Check sheet for the modelled part. Datum: model origin and axes. Units: mm. A direction names the side the tool comes from. Coordinates: 2 decimals unless noted, no trailing zeros. Loops run counter-clockwise (first coordinate to the right, second up) from the corner with the lowest first, then second, coordinate; pieces in that order, holes last.
```python
from build123d import *

# Parameters (mm, degrees)
ESQUISSE1_W                  = 100
ESQUISSE1_H                  = 100
BOSS_EXTRU_1_DEPTH           = 8
ESQUISSE2_W                  = 60.2
ESQUISSE2_H                  = 8.2
ENL_V_MAT_EXTRU_1_DEPTH      = 5
CONG_1_R                     = 5
ENL_V_MAT_EXTRU_2_DEPTH      = 5
ESQUISSE4_R                  = 2.25
ENL_V_MAT_EXTRU_3_DEPTH      = 6
ENL_V_MAT_EXTRU_3_DEPTH_BACK = 4


with BuildPart() as part:
    # Esquisse1 → Boss.-Extru.1 (new body)
    with BuildSketch(Plane.XY):
        with Locations((50, 50)):
            Rectangle(ESQUISSE1_W, ESQUISSE1_H)
    extrude(amount=BOSS_EXTRU_1_DEPTH)

    # Esquisse2 → Enlèv. mat.-Extru.1 (cut)
    with BuildSketch(Plane.XY.offset(8)):
        with Locations((50, 38.9)):
            Rectangle(ESQUISSE2_W, ESQUISSE2_H)
    extrude(amount=-ENL_V_MAT_EXTRU_1_DEPTH, mode=Mode.SUBTRACT)

    # Congé1
    cong_1_edges = [part.edges().sort_by_distance(p)[0] for p in [
        (0, 100, 4),
        (100, 100, 4),
        (100, 0, 4),
        (0, 0, 4),
    ]]
    fillet(cong_1_edges, radius=CONG_1_R)

    # Esquisse3 → Enlèv. mat.-Extru.2 (cut)
    with BuildSketch(Plane.XY.offset(8)):
        with BuildLine():
            Line((77.213483043, 43), (80.1, 40.113483043))
            ThreePointArc((80.1, 40.113483043), (80.241421356, 43.141421356), (77.213483043, 43))
        make_face()
        with BuildLine():
            Line((77.213483043, 34.8), (80.1, 37.686516957))
            ThreePointArc((80.1, 37.686516957), (80.241421356, 34.658578644), (77.213483043, 34.8))
        make_face()
        with BuildLine():
            Line((22.786516957, 34.8), (19.9, 37.686516957))
            ThreePointArc((19.9, 37.686516957), (19.758578644, 34.658578644), (22.786516957, 34.8))
        make_face()
        with BuildLine():
            Line((22.786516957, 43), (19.9, 40.113483043))
            ThreePointArc((19.9, 40.113483043), (19.758578644, 43.141421356), (22.786516957, 43))
        make_face()
    extrude(amount=-ENL_V_MAT_EXTRU_2_DEPTH, mode=Mode.SUBTRACT)

    # Esquisse4 → Enlèv. mat.-Extru.3 (cut, two sides)
    with BuildSketch(Plane.XY.offset(3)) as enl_v_mat_extru_3_sk:
        with Locations((50, 38.9)):
            Circle(ESQUISSE4_R)
        with Locations((70, 38.9)):
            Circle(ESQUISSE4_R)
        with Locations((30, 38.9)):
            Circle(ESQUISSE4_R)
    extrude(amount=ENL_V_MAT_EXTRU_3_DEPTH, mode=Mode.SUBTRACT)
    extrude(enl_v_mat_extru_3_sk.sketch, amount=-ENL_V_MAT_EXTRU_3_DEPTH_BACK, mode=Mode.SUBTRACT)


solid = part.part
```
1) Section check C-C on z = 5.25. Enter the section's corners in (x, y).
Answer sheet:
outline: (0, 5) arc R5 ccw to (5, 0) - (95, 0) arc R5 ccw to (100, 5) - (100, 95) arc R5 ccw to (95, 100) - (5, 100) arc R5 ccw to (0, 95) - close; hole (19.9, 37.69) arc R2.05 ccw (long way) to (22.79, 34.8) - (77.21, 34.8) arc R2.05 ccw (long way) to (80.1, 37.69) - (80.1, 40.11) arc R2.05 ccw (long way) to (77.21, 43) - (22.79, 43) arc R2.05 ccw (long way) to (19.9, 40.11) - close
2) Set-up check for faces 5 (the cylindrical face through (80.27, 43.11, 5.54)), 6 (the flat face through (49, 0, 4)): record each of +Z, -Z, +X, -X, +Y, -Y from which the full face is reachable in a straight line by a thin tool's end or side.
Answer sheet:
face 5: +Z
face 6: +Z, -Z, +X, -X, -Y
3) Scan lines: line 1 (Y direction, x = 50, z = 1.7); line 2 (Y direction, x = 69, z = 6); line 3 (X direction, y = 40.5, z = 2.25). Record each from-to range of solid material in increasing order.
Answer sheet:
line 1: y = 0 to 36.65, 41.15 to 100
line 2: y = 0 to 34.8, 43 to 100
line 3: x = 0 to 28.42, 31.58 to 48.42, 51.58 to 68.42, 71.58 to 100
4) Section check A-A on x = 70. Enter the section's corners in (y, z).
Answer sheet:
outline: (0, 0) - (36.65, 0) - (36.65, 3) - (34.8, 3) - (34.8, 8) - (0, 8) - close; (41.15, 0) - (100, 0) - (100, 8) - (43, 8) - (43, 3) - (41.15, 3) - close
5) Depth check by flat-ended pin: pin 1 (3.5 mm diameter, centred on x = 70, y = 38.9, fed in from +Z); pin 2 (5 mm diameter, centred on x = 49.5, y = 37.5, fed in from +Z); pin 3 (3.5 mm diameter, centred on x = 21.21, y = 41.69, fed in from -Z). Enter the tip coordinate at first touch or a pass-through.
Answer sheet:
pin 1: passes through
pin 2: stops at z = 3
pin 3: stops at z = 0
6) Section check B-B on y = 38.9. Enter the section's corners in (x, z).
Answer sheet:
outline: (0, 0) - (27.75, 0) - (27.75, 3) - (19.9, 3) - (19.9, 8) - (0, 8) - close; (32.25, 0) - (47.75, 0) - (47.75, 3) - (32.25, 3) - close; (52.25, 0) - (67.75, 0) - (67.75, 3) - (52.25, 3) - close; (72.25, 0) - (100, 0) - (100, 8) - (80.1, 8) - (80.1, 3) - (72.25, 3) - close
7) Mould release check, pull along X, two halves, no side actions. Record for faces 1 (the flat face through (100, 49, 4)), 2 (the cylindrical face through (71.038, 36.904, 1.521)), 3 (the flat face through (0, 49, 4)), 4 (the flat face through (50, 42, 3)): +X half, -X half, draft (parallel to the pull), parting line (faces both ways), or undercut.
Answer sheet:
face 1: +X half
face 2: undercut
face 3: -X half
face 4: undercut
8) Section check D-D on x = 59. Enter the section's corners in (y, z).
Answer sheet:
outline: (0, 0) - (100, 0) - (100, 8) - (43, 8) - (43, 3) - (34.8, 3) - (34.8, 8) - (0, 8) - close
